Input: part model. Units: mm. Frame: model coordinates. Face numbers are marked on the shaded views. A direction names the side the tool comes from. Coordinates: 2 decimals unless noted, no trailing zeros. Order: outer loops, then holes, each group sorted by start corner. A loop starts at its lowest first (then second) coordinate and runs counter-clockwise, first axis right, second up. Notation, with made-up numbers: (31, -35.5) -> (82, -35.5) arc R20 ccw to (82, -27.5) -> close; hole circle Ø5 at (-33.5, 22.25). An arc over 180 degrees is marked (long way). Write each question's results on one line, items separated by ' | '.
```python
from build123d import *

# Parameters (mm, degrees)
ESQUISSE1_W             = 85
ESQUISSE1_H             = 56
BOSS_EXTRU_1_DEPTH      = 2
D_GAGEMENT_M21_D        = 2.4
ESQUISSE4_W             = 50
ESQUISSE4_H             = 5
BOSS_EXTRU_3_DEPTH      = 2.5
ESQUISSE6_W             = 49
ESQUISSE6_H             = 3.2
BOSS_EXTRU_5_DEPTH      = 6.2
ESQUISSE3_W             = 22
ESQUISSE3_H             = 16.2
ESQUISSE3_W_2           = 17.6
ESQUISSE3_H_2           = 15
BOSS_EXTRU_2_DEPTH      = 16.3
ESQUISSE7_W             = 12
ESQUISSE7_H             = 5.2
ESQUISSE7_W_2           = 10
ESQUISSE7_H_2           = 1.7
ENL_V_MAT_EXTRU_1_DEPTH = 12
ESQUISSE5_W             = 9
ESQUISSE5_H             = 8.2
ESQUISSE5_W_2           = 7.1
BOSS_EXTRU_4_DEPTH      = 3.6
ESQUISSE8_W             = 7
ESQUISSE8_H             = 15
ESQUISSE8_W_2           = 2.7
ESQUISSE8_H_2           = 22
BOSS_EXTRU_6_DEPTH      = 5.5
ESQUISSE9_W             = 15.5
ESQUISSE9_H             = 12.2
BOSS_EXTRU_7_DEPTH      = 1.5
CONG_1_R                = 3


with BuildPart() as part:
    # Esquisse1 → Boss.-Extru.1 (new body)
    with BuildSketch(Plane(origin=(0, 0, 0), x_dir=(1, 0, 0), z_dir=(0, 1, 0))):
        Rectangle(ESQUISSE1_W, ESQUISSE1_H)
    extrude(amount=BOSS_EXTRU_1_DEPTH)

    # Dégagement M21 (through all)
    with Locations(Plane(origin=(-39, 2, -24.5), x_dir=(0, 0, 1), z_dir=(0, 1, 0))):
        with Locations((0, 0), (49, 0), (0, 58), (49, 58)):
            Hole(D_GAGEMENT_M21_D / 2)

    # Esquisse4 → Boss.-Extru.3 (add)
    with BuildSketch(Plane(origin=(0, 2, 0), x_dir=(1, 0, 0), z_dir=(0, 1, 0))):
        with Locations((-10.795881497, 24.765474627)):
            Rectangle(ESQUISSE4_W, ESQUISSE4_H)
    extrude(amount=BOSS_EXTRU_3_DEPTH)

    # Esquisse6 → Boss.-Extru.5 (add)
    with BuildSketch(Plane(origin=(0, 4.5, 0), x_dir=(1, 0, 0), z_dir=(0, 1, 0))):
        with Locations((-10.795881497, 24.765474627)):
            Rectangle(ESQUISSE6_W, ESQUISSE6_H)
    extrude(amount=BOSS_EXTRU_5_DEPTH)

    # Esquisse3 → Boss.-Extru.2 (add)
    with BuildSketch(Plane(origin=(0, 2, 0), x_dir=(1, 0, 0), z_dir=(0, 1, 0))):
        with Locations((34.7, 17.4)):
            Rectangle(ESQUISSE3_W, ESQUISSE3_H)
        with Locations((36.9, -18.5)):
            Rectangle(ESQUISSE3_W_2, ESQUISSE3_H_2)
        with Locations((36.9, -0.85)):
            Rectangle(ESQUISSE3_W_2, ESQUISSE3_H_2)
    extrude(amount=BOSS_EXTRU_2_DEPTH)

    # Esquisse7 → Enlèv. mat.-Extru.1 (cut)
    # profile 1 of 5: a face of its own
    with BuildSketch(Plane(origin=(45.7, 0, 0), x_dir=(0, 0, -1), z_dir=(1, 0, 0))):
        Polygon((23.4, 15.15), (11.4, 15.15), (11.4, 6.785251797), (15.080363944, 6.785251797), (15.080363944, 5.15), (19.719636056, 5.15), (19.719636056, 6.785251797), (23.4, 6.785251797), align=None)
    # profile 2 of 5: a face of its own
    with BuildSketch(Plane(origin=(45.7, 0, 0), x_dir=(0, 0, -1), z_dir=(1, 0, 0))):
        with Locations((-18.45, 14.7)):
            Rectangle(ESQUISSE7_W, ESQUISSE7_H)
        with Locations((-18.45, 15.45)):
            Rectangle(ESQUISSE7_W_2, ESQUISSE7_H_2, mode=Mode.SUBTRACT)
    # profile 3 of 5: a face of its own
    with BuildSketch(Plane(origin=(45.7, 0, 0), x_dir=(0, 0, -1), z_dir=(1, 0, 0))):
        with Locations((-0.85, 14.7)):
            Rectangle(ESQUISSE7_W, ESQUISSE7_H)
        with Locations((-0.85, 15.45)):
            Rectangle(ESQUISSE7_W_2, ESQUISSE7_H_2, mode=Mode.SUBTRACT)
    # profile 4 of 5: a face of its own
    with BuildSketch(Plane(origin=(45.7, 0, 0), x_dir=(0, 0, -1), z_dir=(1, 0, 0))):
        with Locations((-18.45, 6.55)):
            Rectangle(ESQUISSE7_W, ESQUISSE7_H)
        with Locations((-18.45, 7.3)):
            Rectangle(ESQUISSE7_W_2, ESQUISSE7_H_2, mode=Mode.SUBTRACT)
    # profile 5 of 5: a face of its own
    with BuildSketch(Plane(origin=(45.7, 0, 0), x_dir=(0, 0, -1), z_dir=(1, 0, 0))):
        with Locations((-0.85, 6.55)):
            Rectangle(ESQUISSE7_W, ESQUISSE7_H)
        with Locations((-0.85, 7.3)):
            Rectangle(ESQUISSE7_W_2, ESQUISSE7_H_2, mode=Mode.SUBTRACT)
    extrude(amount=-ENL_V_MAT_EXTRU_1_DEPTH, mode=Mode.SUBTRACT)

    # Esquisse5 → Boss.-Extru.4 (add)
    with BuildSketch(Plane(origin=(0, 2, 0), x_dir=(1, 0, 0), z_dir=(0, 1, 0))):
        with Locations((-31.2, -25.3)):
            Rectangle(ESQUISSE5_W, ESQUISSE5_H)
        with Locations((-16.25, -25.3)):
            Rectangle(ESQUISSE5_W_2, ESQUISSE5_H)
        with Locations((-2.25, -25.3)):
            Rectangle(ESQUISSE5_W_2, ESQUISSE5_H)
    extrude(amount=BOSS_EXTRU_4_DEPTH)

    # Esquisse8 → Boss.-Extru.6 (add)
    with BuildSketch(Plane(origin=(0, 2, 0), x_dir=(1, 0, 0), z_dir=(0, 1, 0))):
        with Locations((11.2, -23)):
            Rectangle(ESQUISSE8_W, ESQUISSE8_H)
        with Locations((3.65, -16)):
            Rectangle(ESQUISSE8_W_2, ESQUISSE8_H_2)
        with Locations((-38.45, 0)):
            Rectangle(ESQUISSE8_W_2, ESQUISSE8_H_2)
    extrude(amount=BOSS_EXTRU_6_DEPTH)

    # Esquisse9 → Boss.-Extru.7 (add)
    with BuildSketch(Plane.XZ):
        with Locations((-37.25, 0)):
            Rectangle(ESQUISSE9_W, ESQUISSE9_H)
    extrude(amount=BOSS_EXTRU_7_DEPTH)

    # Congé1
    # the kernel refuses this fillet: 3 mm, written as the material it takes off along each edge
    with BuildSketch(Plane(origin=(42.5, -7.5, 28), x_dir=(0, 0, -1), z_dir=(0, 1, 0)), Plane(origin=(42.5, -7.5, -28), x_dir=(-1, 0, 0), z_dir=(0, 1, 0))) as cong_1_piece_1:
        with BuildLine():
            CenterArc((CONG_1_R, CONG_1_R), CONG_1_R, 180, 90)
            Line((0, CONG_1_R), (0, 0))
            Line((0, 0), (CONG_1_R, 0))
        make_face()
    extrude(amount=9.5, mode=Mode.SUBTRACT)
    with BuildSketch(Plane(origin=(-42.5, -7.5, 28), x_dir=(0, 0, -1), z_dir=(0, 1, 0)), Plane(origin=(-42.5, -7.5, -28), x_dir=(1, 0, 0), z_dir=(0, 1, 0))) as cong_1_piece_2:
        with BuildLine():
            CenterArc((CONG_1_R, -CONG_1_R), CONG_1_R, 90, 90)
            Line((0, -CONG_1_R), (0, 0))
            Line((0, 0), (CONG_1_R, 0))
        make_face()
    extrude(amount=17, mode=Mode.SUBTRACT)


solid = part.part
```
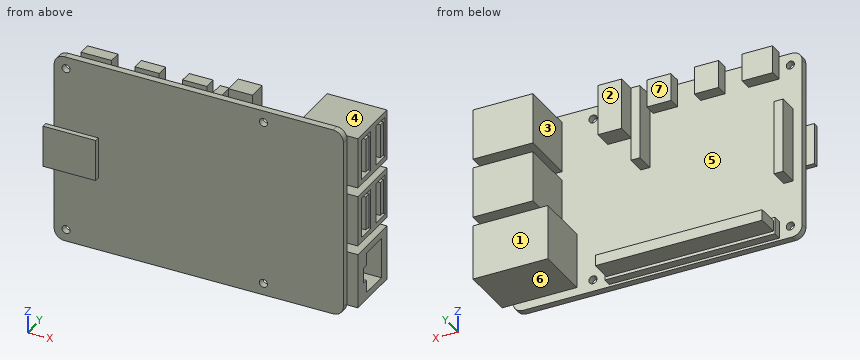
(1) Line query: line 1 along X through (y, z) = (1, -24.5); line 2 along Z through (x, y) = (38, 10.25); line 3 along X through (y, z) = (4.75, 5.5). Output: solid intervals per line, ascending. Write a range as from..to.
Return value:
line 1: -42.5..-40.2, -37.8..17.8, 20.2..42.5 | line 2: -25.5..-23.4, -11.4..-9.3, -6.65..8.35, 11..26 | line 3: -39.8..-37.1, 2.3..5, 28.1..33.7
(2) Cut plane A-A, the plane y = 13. Return loops of the section in (x, z), plus the area to 3 significant figures.
Return value:
outline: (23.7, -25.5) -> (45.7, -25.5) -> (45.7, -23.4) -> (33.7, -23.4) -> (33.7, -11.4) -> (45.7, -11.4) -> (45.7, -9.3) -> (23.7, -9.3) -> close; (28.1, -6.65) -> (45.7, -6.65) -> (45.7, -5.15) -> (33.7, -5.15) -> (33.7, 6.85) -> (45.7, 6.85) -> (45.7, 8.35) -> (28.1, 8.35) -> close; (28.1, 11) -> (45.7, 11) -> (45.7, 12.45) -> (33.7, 12.45) -> (33.7, 24.45) -> (45.7, 24.45) -> (45.7, 26) -> (28.1, 26) -> close | area: 452 mm2
(3) Cut plane B-B, the plane x = 19. Return loops of the section in (y, z), plus the area to 3 significant figures.
Return value:
outline: (0, -28) -> (2, -28) -> (2, -25.7) -> (0, -25.7) -> close; (0, -23.3) -> (2, -23.3) -> (2, 23.3) -> (0, 23.3) -> close; (0, 25.7) -> (2, 25.7) -> (2, 28) -> (0, 28) -> close | area: 102 mm2
(4) Pin query (flat end, axial travel): P1, Ø3, axis at x = -39, z = 24.5, coming from the -Y side; P2, Ø1.6, axis at y = 0.5, z = -3.5, coming from the +X side; P3, Ø3, axis at x = 32.5, y = 13.5, coming from the -Z side; P4, Ø2, axis at y = 3.5, z = -26, coming from the +X side. Return the tip coordinate at first contact, or that it passes through.
Return value:
P1: y = 0 | P2: x = 42.5 | P3: z = -25.5 | P4: x = 45.7
(5) Mould query, pull axis Z, two halves, no side actions, for the marked faces 4, 5, 6 and 7. Classes: +Z half, -Z half, draft (parallel to the pull), parting line (faces both ways), or undercut.
Return value:
face 4: +Z half | face 5: undercut | face 6: -Z half | face 7: draft
(6) Reachability of the marked faces 1, 2 and 3 from +Z, -Z, +X, -X, +Y, -Y: full face, straight path, thin tool, end or side. Return the list, or none.
Return value:
face 1: +Z, -Z, +X, -X, +Y | face 2: +Z, -X, +Y | face 3: +Z, +Y
